Verification items for the finished model (mm, model axes). Round coordinates to 2 decimals unless told otherwise and drop trailing zeros. Write each loop counter-clockwise with the first axis right and the second up, starting at its lowest first coordinate (ties: lowest second). Pieces come first, ordered by that corner, then holes. Notation, with made-up numbers: M -23.75,65 L 8.25,65 A24 ccw 8.25,91 Z; hole C 35.5,-18 d9. An arc over 180 degrees is marked long. One line per item, written item: value. Start each with the question number.
Item 1: Section check A-A, the plane z = 2.25. Record the cut outline in (x, y) (3 decimals), then the cut area to 3 significant figures.
Item 2: Section check B-B, the plane y = -27.5. Record the cut outline in (x, z).
Item 3: Thickness scan on probe 1 along Y at (x, z) = (17, 22.5); probe 2 along Y at (x, z) = (16, 21.75); probe 3 along Z at (x, y) = (-8, -38.5). Record the ranges inside material, lowest first. Write a range as from..to.
Item 4: Section check C-C, the plane z = 23.5. Record the cut outline in (x, y) (3 decimals).
from build123d import *

# Parameters (mm, degrees)
F0_W     = 65.410413
F0_H     = 64.301759
F1_DEPTH = 25.4
F3_R     = 5.08
F4_D     = 6.35


with BuildPart() as f1:
    # F0 (on Top) → F1 (new body)
    with BuildSketch(Plane.XY):
        with Locations((10.90173, -10.716959)):
            Rectangle(F0_W, F0_H)
    extrude(amount=F1_DEPTH)

    # F3
    f3_edges = [f1.edges().sort_by_distance(p)[0] for p in [
        (10.901731, 21.43392, 25.4),
        (-21.803476, 21.43392, 12.7),
        (10.901731, 21.43392, 0),
        (-21.803476, -10.71696, 0),
        (10.901731, -42.867839, 0),
        (43.606937, -10.71696, 0),
    ]]
    fillet(f3_edges, radius=F3_R)

    # F4 (through all)
    with Locations(Plane(origin=(0, 0, 0), x_dir=(1, 0, 0), z_dir=(0, 0, -1))):
        with Locations((-21.803476, 27.994836)):
            Hole(F4_D / 2)


solid = f1.part
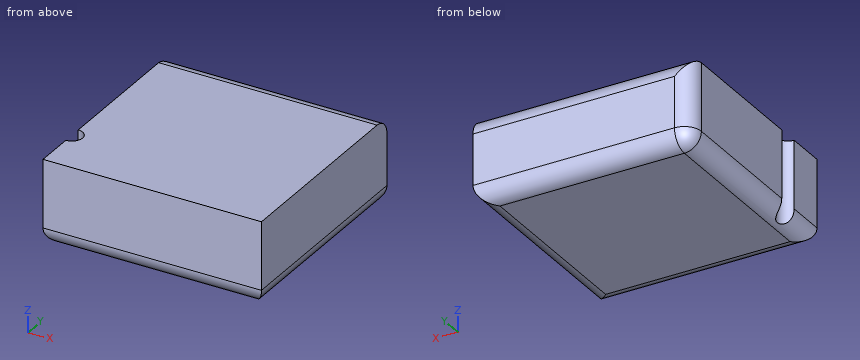
Response values:
1. outline: M -20.942,-42.007 L 42.746,-42.007 L 42.746,20.573 L -16.723,20.573 A4.219 ccw -20.942,16.354 L -20.942,-24.939 A3.175 cw -20.942,-31.051 Z
1. area: 3,970 mm2
2. outline: M -18.67,0.39 A5.08 ccw -16.72,0 L 38.53,0 A5.08 ccw 43.61,5.08 L 43.61,25.4 L -18.67,25.4 Z
3. probe 1: y = -42.87..20.94
3. probe 2: y = -42.87..21.23
3. probe 3: z = 0.05..25.4
4. outline: M -21.803,-42.868 L 43.607,-42.868 L 43.607,20.315 L -19.903,20.315 A5.08 ccw -21.803,16.354 L -21.803,-24.82 A3.175 cw -21.803,-31.17 Z
